Geometry: final body of the model. Coordinates: model frame, mm. A direction names the side the tool comes from. Round coordinates to 2 decimals unless told otherwise and drop trailing zeros. Loops run counter-clockwise (first coordinate to the right, second up) from the corner with the lowest first, then second, coordinate; pieces in that order, holes last. Notation, with made-up numbers: M -21.75,86.25 L -9.75,86.25 A25 ccw -9.75,115.25 Z; hole C 56.5,54.5 d4. An arc over 180 degrees is marked long. Write each question's results on one line, items separated by ' | '.
```python
from build123d import *

# Parameters (mm, degrees)
EXTRUDE_THIN1_DEPTH  = 180.34
LPATTERN1_COUNT      = 2
LPATTERN1_PITCH      = 20.32
LPATTERN1_COUNT_DIR2 = 9
LPATTERN1_PITCH_DIR2 = 17.78


with BuildPart() as part:
    # Sketch1 → Extrude-Thin1 (new body)
    with BuildSketch(Plane.XY):
        Polygon((0, 0), (11.202174456, 24.023140647), (20.203364855, -0.707426722), (17.816545598, -1.576157886), (10.912657758, 17.392118062), (2.302021779, -1.073450385), align=None)
    extrude_thin1 = extrude(amount=-EXTRUDE_THIN1_DEPTH)

    # LPattern1: Extrude-Thin1 2 × 9, 9 skipped
    with Locations(*[(j * LPATTERN1_PITCH_DIR2, i * LPATTERN1_PITCH, 0) for i in range(LPATTERN1_COUNT) for j in range(LPATTERN1_COUNT_DIR2) if (i, j) not in ((0, 0), (1, 0), (1, 1), (1, 2), (1, 3), (1, 4), (1, 5), (1, 6), (1, 7), (1, 8))]):
        add(extrude_thin1)


solid = part.part
```
1. Section B-B (x = 104.5). Output: boundary loops of the cut face in (y, z).
Answer key:
outline: M 4.51,-180.34 L 11.94,-180.34 L 11.94,0 L 4.51,0 Z
2. Ray query, probe 1 along Y at (x, z) = (96.5, -42); probe 2 along Y at (x, z) = (128, -162.5). Return the intervals inside material, ascending.
Answer key:
probe 1: y = 10.29 to 16.3 | probe 2: y = 1.58 to 7.59
3. Access query for faces 3 (the face through (148.38, 13.17, -88.91)), 4 (the face through (49.97, 7.78, -88.91)). Directions: +Z, -Z, +X, -X, +Y, -Y. A direction counts if a zero-diameter tool reaches every point of the face in a straight line with its end or side. Return the directions, or none.
Answer key:
face 3: +Z, -Z, +Y | face 4: +Z, -Z, -Y
4. Pin query (flat end, axial travel): P1, Ø4, axis at y = 12.5, z = -156.5, coming from the +X side; P2, Ø1.5, axis at x = 74, z = -69.5, coming from the -Y side; P3, Ø5, axis at x = 117.5, y = 10.5, coming from the +Z side; P4, Ø3, axis at x = 90.5, z = -84.5, coming from the +Y side. Return the tip coordinate at first contact, or that it passes through.
Answer key:
P1: stops at x = 158.36 | P2: stops at y = -1.07 | P3: stops at z = 0 | P4: stops at y = 6.65
5. Section A-A (y = 6.5). Count the separate pieces of the cut face and the enclosed holes in it, then the cut area to 3 significant figures.
Answer key:
separate pieces: 18 | enclosed holes: 0 | area: 8,940 mm²
6. Draft query along X for faces 1 (the face through (87.6, 8.4, -180.34)), 2 (the face through (60.01, 8.29, -88.91)). Return one class per face: pulls with the +X half, pulls with the -X half, needs draft (parallel to the pull), parting line crosses it, or undercut.
Answer key:
face 1: needs draft | face 2: undercut
